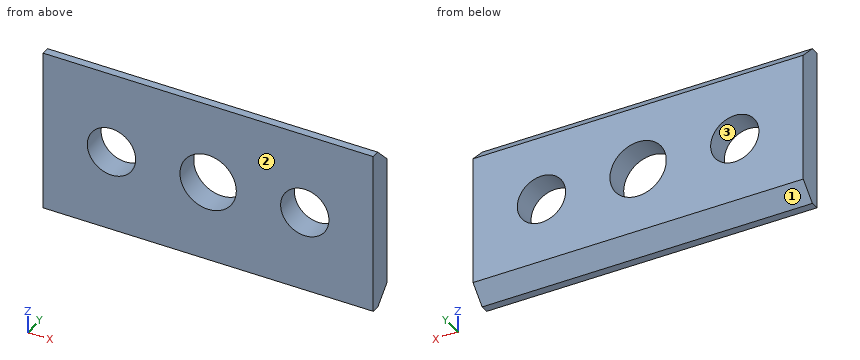
from build123d import *

# Parameters (mm, degrees)
SKETCH1_W           = 41
SKETCH1_H           = 20
BOSS_EXTRUDE1_DEPTH = 3
SKETCH7_R           = 3
SKETCH7_R_2         = 3.5
HOLES_DEPTH         = 4
CHAMFER1_SIZE       = 2


with BuildPart() as part:
    # Sketch1 → Boss-Extrude1 (new body)
    with BuildSketch(Plane(origin=(0, 0, 0), x_dir=(1, 0, 0), z_dir=(0, 1, 0))):
        with Locations((20.5, 10)):
            Rectangle(SKETCH1_W, SKETCH1_H)
    extrude(amount=-BOSS_EXTRUDE1_DEPTH)

    # Sketch7 → holes (cut, through all)
    with BuildSketch(Plane(origin=(0, 0, 0), x_dir=(1, 0, 0), z_dir=(0, 1, 0))):
        with Locations((8.5, 10)):
            Circle(SKETCH7_R)
        with Locations((32.5, 10)):
            Circle(SKETCH7_R)
        with Locations((20.5, 10)):
            Circle(SKETCH7_R_2)
    extrude(amount=-HOLES_DEPTH, mode=Mode.SUBTRACT)

    # Chamfer1
    chamfer1_edges = [part.edges().sort_by_distance(p)[0] for p in [
        (20.5, 0, 0),
        (20.5, 0, -20),
    ]]
    chamfer(chamfer1_edges, length=CHAMFER1_SIZE)


solid = part.part
For this review, take the finished solid that the model builds, in its own axes (mm). Face numbers are marked on the shaded views. Give positions to 0.01 mm unless a question says otherwise; leave off trailing zeros. Loops run counter-clockwise (first coordinate to the right, second up) from the corner with the lowest first, then second, coordinate; pieces in that order, holes last. Notation, with made-up numbers: M -23,51 L 7,51 A14 ccw 7,67 Z; hole C -38,60.25 d4. An arc over 180 degrees is marked long. Put each result on its own line as item: value. Start each with the question number.
(1) Add section D-D, the plane x = 15. Write out the cut boundary in (y, z).
(2) For pin 1 (1.5 mm diameter, centred on y = -1.5, z = -11, fed in from -X); pin 2 (6.5 mm diameter, centred on x = 20.5, z = -10, fed in from +Y), all flat-tipped, find the tip position at first contact; note any pin that passes through.
(3) Add section C-C, the plane x = 32.5. Write out the cut boundary in (y, z), then the cut area to 3 significant figures.
(4) Wall thickness on L1, parallel to X at y = -2.15, z = -10; L2, parallel to Z at x = 20.5, y = -2.15; L3, parallel to X at y = -1.65, z = -12.5: over which ranges is each line inside the solid? List them lowest first.
(5) The part is to be moulded in two halves that separate along Z. For the marked faces 1, 2 and 3, say which applies: +Z half, -Z half, draft (parallel to the pull), parting line (faces both ways), or undercut.
(6) Add section B-B, the plane z = -10. Write out the cut boundary in (x, y), then the cut area to 3 significant figures.
(7) Add section A-A, the plane y = -0.4. Write out the cut boundary in (x, z), then the cut area to 3 significant figures.
Result:
1. outline: M -3,-20 L -2,-20 L 0,-18 L 0,-2 L -2,0 L -3,0 Z
2. pin 1: stops at x = 0
2. pin 2: passes through
3. outline: M -3,-20 L -2,-20 L 0,-18 L 0,-13 L -3,-13 Z; M -3,-7 L 0,-7 L 0,-2 L -2,0 L -3,0 Z
3. area: 38.0 mm^2
4. L1: x = 0 to 5.5, 11.5 to 17, 24 to 29.5, 35.5 to 41
4. L2: z = -20 to -13.5, -6.5 to 0
4. L3: x = 0 to 6.84, 10.16 to 18.05, 22.95 to 30.84, 34.16 to 41
5. face 1: -Z half
5. face 2: draft
5. face 3: undercut
6. outline: M 0,-3 L 5.5,-3 L 5.5,0 L 0,0 Z; M 11.5,-3 L 17,-3 L 17,0 L 11.5,0 Z; M 24,-3 L 29.5,-3 L 29.5,0 L 24,0 Z; M 35.5,-3 L 41,-3 L 41,0 L 35.5,0 Z
6. area: 66.0 mm^2
7. outline: M 0,-18.4 L 41,-18.4 L 41,-1.6 L 0,-1.6 Z; hole C 8.5,-10 d6; hole C 20.5,-10 d7; hole C 32.5,-10 d6
7. area: 594 mm^2
